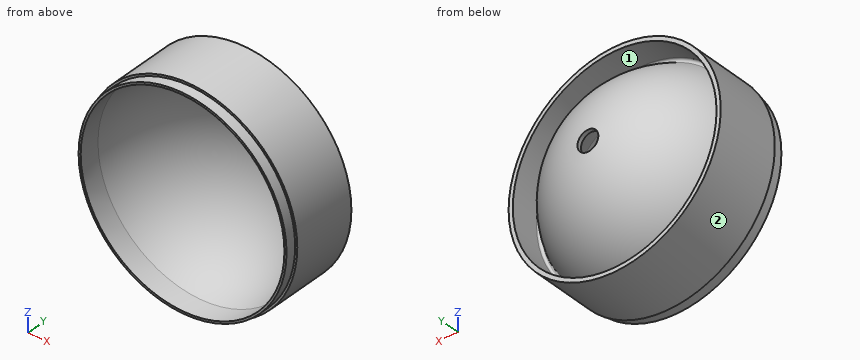
from build123d import *

# Parameters (mm, degrees)
SKETCH3_R          = 12.5
CUT_EXTRUDE1_DEPTH = 1000


with BuildPart() as part:
    # Sketch2 → Revolve1 (revolve)
    with BuildSketch(Plane.XY):
        with BuildLine():
            Line((127, 900), (127, 965.730277379))
            Line((127, 965.730277379), (122, 965.730277379))
            Line((122, 965.730277379), (122, 931.460554757))
            ThreePointArc((122, 931.460554757), (120.042413497, 929.02010652), (117.235369921, 930.401569108))
            ThreePointArc((117.235369921, 930.401569108), (69.478517997, 984.769156682), (0, 1005))
            Line((0, 1005), (0, 1000))
            ThreePointArc((0, 1000), (78.873316147, 971.805445699), (122, 900))
            Line((122, 900), (122, 875))
            Line((122, 875), (124.5, 875))
            Line((124.5, 875), (124.5, 887.5))
            Line((124.5, 887.5), (127, 887.5))
            Line((127, 887.5), (127, 900))
        make_face()
    revolve(axis=Axis((0, 0, 0), (0, 1, 0)))

    # Sketch3 → Cut-Extrude1 (cut)
    with BuildSketch(Plane.XZ.offset(-875)):
        Circle(SKETCH3_R)
    extrude(amount=-CUT_EXTRUDE1_DEPTH, mode=Mode.SUBTRACT)


solid = part.part
Check sheet for the modelled part. Datum: model origin and axes. Units: mm. Face numbers are marked on the shaded views. Give positions to 0.01 mm unless a question says otherwise; leave off trailing zeros. Write each loop counter-clockwise with the first axis right and the second up, starting at its lowest first coordinate (ties: lowest second). Pieces come first, ordered by that corner, then holes. Notation, with made-up numbers: (65.5, 72) -> (110.5, 72) arc R22 cw to (110.5, 110) -> close; hole circle Ø4 at (73, 64.25). An arc over 180 degrees is marked (long way). One line per item, written item: value. Start each with the question number.
Item 1: Section check D-D on y = 915.5. Record the cut outline in (x, z), then the cut area to 3 significant figures.
Item 2: Section check B-B on x = 0. Record the cut outline in (y, z).
Item 3: Material ranges on probe 1 along Z at (x, y) = (-33, 941); probe 2 along Z at (x, y) = (47.5, 931.5); probe 3 along X at (y, z) = (951.5, -73.5), recorded low to high. Write a range as from..to.
Item 4: Draft check along Z on the marked faces 1 and 2. Enter one of: +Z half, -Z half, draft (parallel to the pull), parting line (faces both ways), or undercut.
Item 5: Section check C-C on y = 884. Record the cut outline in (x, z), then the cut area to 3 significant figures.
Item 6: Gauge pin test, flat ends, axial feed: pin 1 (12 mm diameter, centred on x = 100.5, y = 903, fed in from -Z); pin 2 (10 mm diameter, centred on x = 97, z = 18.5, fed in from +Y); pin 3 (3 mm diameter, centred on x = 31, y = 938, fed in from +Z). Record the tip position at first contact, or that the pin passes through.
Item 7: Section check A-A on z = 0. Record the cut outline in (x, y), then the cut area to 3 significant figures.
Results list:
1. outline: circle Ø254 at (0, 0); hole circle Ø235.68 at (0, 0)
1. area: 7,040 mm²
2. outline: (875, -124.5) -> (887.5, -124.5) -> (887.5, -127) -> (965.73, -127) -> (965.73, -122) -> (931.46, -122) arc R2.5 cw to (930.4, -117.24) arc R129.42 ccw to (1004.39, -12.5) -> (999.37, -12.5) arc R124.42 cw to (900, -122) -> (875, -122) -> close; (875, 122) -> (900, 122) arc R124.42 cw to (999.37, 12.5) -> (1004.39, 12.5) arc R129.42 ccw to (930.4, 117.24) arc R2.5 cw to (931.46, 122) -> (965.73, 122) -> (965.73, 127) -> (887.5, 127) -> (887.5, 124.5) -> (875, 124.5) -> close
3. probe 1: -122.64..-117.45, -106.68..-100.56, 100.56..106.68, 117.45..122.64
3. probe 2: -117.78..-112.37, -106.61..-100.48, 100.48..106.61, 112.37..117.78
3. probe 3: -103.57..-97.37, -74.72..-65.68, 65.68..74.72, 97.37..103.57
4. face 1: undercut
4. face 2: parting line
5. outline: circle Ø249 at (0, 0); hole circle Ø244 at (0, 0)
5. area: 1,940 mm²
6. pin 1: z = -84.85
6. pin 2: y = 964.8
6. pin 3: z = 123.53
7. outline: (-127, 887.5) -> (-124.5, 887.5) -> (-124.5, 875) -> (-122, 875) -> (-122, 900) arc R124.42 cw to (-12.5, 999.37) -> (-12.5, 1004.39) arc R129.42 ccw to (-117.24, 930.4) arc R2.5 cw to (-122, 931.46) -> (-122, 965.73) -> (-127, 965.73) -> close; (12.5, 999.37) arc R124.42 cw to (122, 900) -> (122, 875) -> (124.5, 875) -> (124.5, 887.5) -> (127, 887.5) -> (127, 965.73) -> (122, 965.73) -> (122, 931.46) arc R2.5 cw to (117.24, 930.4) arc R129.42 ccw to (12.5, 1004.39) -> close
7. area: 2,410 mm²
